```python
from build123d import *

# Parameters (mm, degrees)
BOSS_EXTRUDE1_START = -25.4
SKETCH1_W           = 75.4
SKETCH1_H           = 75.4
SKETCH1_R           = 2.025
BOSS_EXTRUDE1_DEPTH = 6.35
SKETCH2_W           = 75.4
SKETCH2_H           = 88.5
SKETCH2_R           = 2.025
BOSS_EXTRUDE2_DEPTH = 6.35
BOSS_EXTRUDE3_START = -37.7
BOSS_EXTRUDE3_DEPTH = 75.4
CUT_EXTRUDE1_DEPTH  = 31.75
FILLET3_R           = 6.35
FILLET4_R           = 3.175


with BuildPart() as part:
    # Sketch1 → Boss-Extrude1 (new body)
    with BuildSketch(Plane(origin=(0, 0, 0), x_dir=(1, 0, 0), z_dir=(0, 1, 0)).offset(BOSS_EXTRUDE1_START)):
        Rectangle(SKETCH1_W, SKETCH1_H)
        with Locations((-25, 25)):
            Circle(SKETCH1_R, mode=Mode.SUBTRACT)
        with Locations((25, 25)):
            Circle(SKETCH1_R, mode=Mode.SUBTRACT)
        with Locations((25, -25)):
            Circle(SKETCH1_R, mode=Mode.SUBTRACT)
        with Locations((-25, -25)):
            Circle(SKETCH1_R, mode=Mode.SUBTRACT)
    extrude(amount=-BOSS_EXTRUDE1_DEPTH)

    # Sketch2 → Boss-Extrude2 (add)
    with BuildSketch(Plane.ZY.offset(37.7)):
        with Locations((0, 12.5)):
            Rectangle(SKETCH2_W, SKETCH2_H)
        with Locations((-25, 44.05)):
            Circle(SKETCH2_R, mode=Mode.SUBTRACT)
        with Locations((-25, -5.95)):
            Circle(SKETCH2_R, mode=Mode.SUBTRACT)
        with Locations((25, -5.95)):
            Circle(SKETCH2_R, mode=Mode.SUBTRACT)
        with Locations((25, 44.05)):
            Circle(SKETCH2_R, mode=Mode.SUBTRACT)
    extrude(amount=BOSS_EXTRUDE2_DEPTH)

    # Sketch3 → Boss-Extrude3 (add)
    with BuildSketch(Plane(origin=(0, 0, 0), x_dir=(-1, 0, 0), z_dir=(0, 0, -1)).offset(BOSS_EXTRUDE3_START)):
        Polygon((-37.7, -25.4), (37.7, 56.75), (37.7, 47.359169269), (-29.08078348, -25.4), align=None)
    extrude(amount=BOSS_EXTRUDE3_DEPTH)

    # Sketch3<2> → Cut-Extrude1 (cut, symmetric)
    with BuildSketch(Plane(origin=(0, 0, 0), x_dir=(-1, 0, 0), z_dir=(0, 0, -1))):
        Polygon((-37.7, -25.4), (37.7, 56.75), (37.7, 47.359169269), (-29.08078348, -25.4), align=None)
    extrude(amount=CUT_EXTRUDE1_DEPTH, both=True, mode=Mode.SUBTRACT)

    # Fillet3
    fillet3_edges = [part.edges().sort_by_distance(p)[0] for p in [
        (-37.7, 47.359169269, -34.725),
        (-37.7, -25.4, 0),
        (29.08078348, -25.4, -34.725),
        (-37.7, 47.359169269, 34.725),
        (29.08078348, -25.4, 34.725),
    ]]
    fillet(fillet3_edges, radius=FILLET3_R)

    # Fillet4
    fillet4_edges = [part.edges().sort_by_distance(p)[0] for p in [
        (21.857054709, -25.4, 31.75),
        (-37.7, 39.204519819, 31.75),
        (21.857054709, -25.4, -31.75),
        (-37.7, 39.204519819, -31.75),
    ]]
    fillet(fillet4_edges, radius=FILLET4_R)


solid = part.part
```
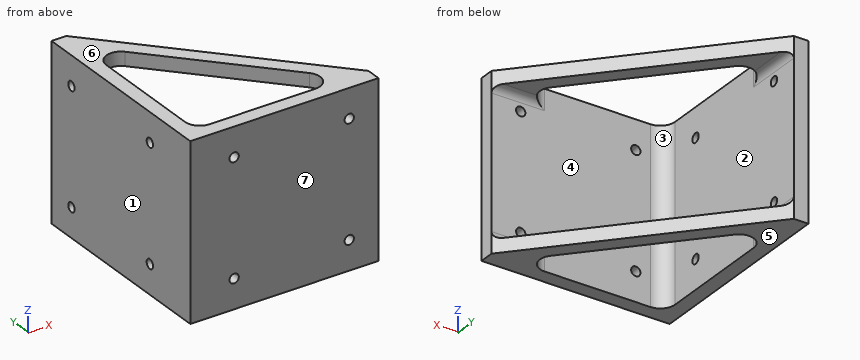
Build history of the part. All positions in model axes, mm. Face numbers are marked on the shaded views. A direction names the side the tool comes from. Coordinates: 2 decimals unless noted, no trailing zeros. Order: outer loops, then holes, each group sorted by start corner. A loop starts at its lowest first (then second) coordinate and runs counter-clockwise, first axis right, second up. Notation, with made-up numbers: M -33.75,38.25 L 11.25,38.25 A19 ccw 11.25,43.25 Z; hole C 66,-6.5 d7. An arc over 180 degrees is marked long. One line per question, with ' | ' between items. Start each with the question number.
1. Wall check: line 1 along X through (y, z) = (-29, -25) (3 decimals); line 2 along Y through (x, z) = (-39, 25) (3 decimals); line 3 along Z through (x, y) = (25, -28) (3 decimals). Give the ranges that are in metal, low to high. Write a range as [from, to].
2. Cut at B-B (x = 25). Write the cut outline in (y, z) (3 decimals).
3. Cut at D-D (z = -14.5). Write the cut outline in (x, y), plus the area to 3 significant figures.
4. Mould opens along Z. For the marked faces 4, 5, 6 and 7 say: +Z half, -Z half, draft (parallel to the pull), parting line (faces both ways), or undercut.
5. Flat gauge pins, fed straight in: P1, Ø3, axis at x = 25, z = -25, coming from the +Y side; P2, Ø4, axis at y = 13.5, z = 16.5, coming from the +X side; P3, Ø6.5, axis at x = -25, z = 25, coming from the -Y side; P4, Ø6.5, axis at x = -25, z = -25, coming from the +Y side. Where does each tip first touch, or does it go through?
6. Tool access for the marked faces 1, 2 and 3: list every direction of +Z, -Z, +X, -X, +Y, -Y with a clear straight run to the whole face (end or side of a thin tool).
7. Cut at C-C (y = 44.05). Write the cut outline in (x, z) (3 decimals).
8. Cut at A-A (z = -25). Write the cut outline in (x, y) (3 decimals).
The answers:
1) line 1: x = [-44.05, -27.025], [-22.975, 22.975], [27.025, 37.7] | line 2: y = [-31.75, -7.975], [-3.925, 42.025], [46.075, 56.75] | line 3: z = [-37.7, -27.025], [-22.975, 22.975], [27.025, 37.7]
2) outline: M -31.75,-37.7 L -11.563,-37.7 L -11.563,-31.75 L -22.225,-31.75 A3.175 cw -25.4,-28.575 L -25.4,-27.025 L -31.75,-27.025 Z; M -31.75,-22.975 L -25.4,-22.975 L -25.4,22.975 L -31.75,22.975 Z; M -31.75,27.025 L -25.4,27.025 L -25.4,28.575 A3.175 cw -22.225,31.75 L -11.563,31.75 L -11.563,37.7 L -31.75,37.7 Z
3) outline: M -44.05,-31.75 L 37.7,-31.75 L 37.7,-25.4 L -31.35,-25.4 A6.35 cw -37.7,-19.05 L -37.7,56.75 L -44.05,56.75 Z | area: 1,050 mm2
4) face 4: undercut | face 5: -Z half | face 6: +Z half | face 7: draft
5) P1: passes through | P2: stops at x = -37.7 | P3: stops at y = -31.75 | P4: stops at y = -25.4
6) face 1: +Z, -Z, -X, +Y, -Y | face 2: none | face 3: +Z, -Z
7) outline: M -44.05,-37.7 L -26.044,-37.7 L -26.044,-31.75 L -34.525,-31.75 A3.175 cw -37.7,-28.575 L -37.7,-27.025 L -44.05,-27.025 Z; M -44.05,-22.975 L -37.7,-22.975 L -37.7,22.975 L -44.05,22.975 Z; M -44.05,27.025 L -37.7,27.025 L -37.7,28.575 A3.175 cw -34.525,31.75 L -26.044,31.75 L -26.044,37.7 L -44.05,37.7 Z
8) outline: M -44.05,-31.75 L -27.025,-31.75 L -27.025,-25.4 L -31.35,-25.4 A6.35 cw -37.7,-19.05 L -37.7,-7.975 L -44.05,-7.975 Z; M -44.05,-3.925 L -37.7,-3.925 L -37.7,42.025 L -44.05,42.025 Z; M -44.05,46.075 L -37.7,46.075 L -37.7,56.75 L -44.05,56.75 Z; M -22.975,-31.75 L 22.975,-31.75 L 22.975,-25.4 L -22.975,-25.4 Z; M 27.025,-31.75 L 37.7,-31.75 L 37.7,-25.4 L 27.025,-25.4 Z
